```python
from build123d import *

# Parameters (mm, degrees)
SKETCH_1_W           = 100.9
SKETCH_1_H           = 40
SKETCH_1_R           = 1.5
EXTRUDE_1_DEPTH      = 6
SKETCH_6_W           = 100.9
SKETCH_6_H           = 10
EXTRUDE_2_DEPTH      = 6
SKETCH_2_W           = 60.5
SKETCH_2_H           = 15
CUT_EXTRUDE_1_DEPTH  = 10
SKETCH_3_R           = 1
CUT_EXTRUDE_2_DEPTH  = 10
SKETCH_4_R           = 1.5
CUT_EXTRUDE_3_DEPTH  = 10
SKETCH_5_R           = 1.5
CUT_EXTRUDE_4_DEPTH  = 10
SKETCH_7_W           = 4
SKETCH_7_H           = 15
CUT_EXTRUDE_5_DEPTH  = 6
CUT_EXTRUDE_6_DEPTH  = 6
FILLET_1_R           = 0.5
FILLET_2_R           = 1
SKETCH_9_W           = 100.9
SKETCH_9_H           = 15
EXTRUDE_3_DEPTH      = 6
SKETCH_10_W          = 16.5
SKETCH_10_H          = 15
CUT_EXTRUDE_7_DEPTH  = 6
SKETCH_11_W          = 6
SKETCH_11_H          = 15
EXTRUDE_4_DEPTH      = 20
SKETCH_12_R          = 2.5
CUT_EXTRUDE_8_DEPTH  = 6
SKETCH_13_R          = 1.5
CUT_EXTRUDE_9_DEPTH  = 6
SKETCH_14_R          = 1.5
CUT_EXTRUDE_10_DEPTH = 6
SKETCH_15_W          = 20
SKETCH_15_H          = 2
EXTRUDE_5_DEPTH      = 6
FILLET_4_R           = 2
FILLET_5_R           = 2
SKETCH_19_R          = 4.5
SKETCH_19_R_2        = 2.5
EXTRUDE_6_DEPTH      = 55.9


with BuildPart() as part:
    # 草图1 → 凸台-拉伸1 (new body)
    with BuildSketch(Plane.XY):
        with Locations((0, 10)):
            Rectangle(SKETCH_1_W, SKETCH_1_H)
        with Locations((42.3, 25)):
            Circle(SKETCH_1_R, mode=Mode.SUBTRACT)
        with Locations((42.3, 5)):
            Circle(SKETCH_1_R, mode=Mode.SUBTRACT)
        with Locations((35.3, 5)):
            Circle(SKETCH_1_R, mode=Mode.SUBTRACT)
        with Locations((35.3, -5)):
            Circle(SKETCH_1_R, mode=Mode.SUBTRACT)
        with Locations(Location((-35.3, -5, 0), (0, 0, 180))):
            Circle(SKETCH_1_R, mode=Mode.SUBTRACT)
        with Locations(Location((-35.3, 5, 0), (0, 0, 180))):
            Circle(SKETCH_1_R, mode=Mode.SUBTRACT)
        with Locations(Location((-42.3, 5, 0), (0, 0, 180))):
            Circle(SKETCH_1_R, mode=Mode.SUBTRACT)
        with Locations(Location((-42.3, 25, 0), (0, 0, 180))):
            Circle(SKETCH_1_R, mode=Mode.SUBTRACT)
    extrude(amount=EXTRUDE_1_DEPTH)

    # 草图6 → 凸台-拉伸2 (add)
    with BuildSketch(Plane.XY.offset(6)):
        with Locations((0, 35)):
            Rectangle(SKETCH_6_W, SKETCH_6_H)
    extrude(amount=-EXTRUDE_2_DEPTH)

    # 草图2 → 切除-拉伸1 (cut)
    with BuildSketch(Plane.XY.offset(6)):
        with Locations((0, -2.5)):
            Rectangle(SKETCH_2_W, SKETCH_2_H)
    extrude(amount=-CUT_EXTRUDE_1_DEPTH, mode=Mode.SUBTRACT)

    # 草图3 → 切除-拉伸2 (cut)
    with BuildSketch(Plane.XY.offset(6)):
        with Locations((-30.25, 5)):
            Circle(SKETCH_3_R)
        with Locations((30.25, 5)):
            Circle(SKETCH_3_R)
    extrude(amount=-CUT_EXTRUDE_2_DEPTH, mode=Mode.SUBTRACT)

    # 草图4 → 切除-拉伸3 (cut)
    with BuildSketch(Plane.XY.offset(6)):
        with Locations((31, 34.5)):
            Circle(SKETCH_4_R)
        with Locations((31, 24.5)):
            Circle(SKETCH_4_R)
        with Locations((-31, 24.5)):
            Circle(SKETCH_4_R)
        with Locations((-31, 34.5)):
            Circle(SKETCH_4_R)
    extrude(amount=-CUT_EXTRUDE_3_DEPTH, mode=Mode.SUBTRACT)

    # 草图5 → 切除-拉伸4 (cut)
    with BuildSketch(Plane.XY.offset(6)):
        with Locations((-15, 12.5)):
            Circle(SKETCH_5_R)
        with Locations((5, 12.5)):
            Circle(SKETCH_5_R)
    extrude(amount=-CUT_EXTRUDE_4_DEPTH, mode=Mode.SUBTRACT)

    # 草图7 → 切除-拉伸5 (cut)
    with BuildSketch(Plane.XY.offset(6)):
        with Locations((36, 27)):
            Rectangle(SKETCH_7_W, SKETCH_7_H)
        with Locations((-36, 27)):
            Rectangle(SKETCH_7_W, SKETCH_7_H)
    extrude(amount=-CUT_EXTRUDE_5_DEPTH, mode=Mode.SUBTRACT)

    # 草图8 → 切除-拉伸6 (cut)
    with BuildSketch(Plane.XY.offset(6)):
        with BuildLine():
            Line((-38, 33.5), (-38, 34.5))
            ThreePointArc((-38, 34.5), (-38.5, 34), (-38, 33.5))
        make_face()
        with BuildLine():
            Line((-34, 34.5), (-34, 33.5))
            ThreePointArc((-34, 33.5), (-33.5, 34), (-34, 34.5))
        make_face()
        with BuildLine():
            Line((-38, 19.5), (-38, 20.5))
            ThreePointArc((-38, 20.5), (-38.5, 20), (-38, 19.5))
        make_face()
        with BuildLine():
            Line((-34, 20.5), (-34, 19.5))
            ThreePointArc((-34, 19.5), (-33.5, 20), (-34, 20.5))
        make_face()
        with BuildLine():
            ThreePointArc((38, 33.5), (38.5, 34), (38, 34.5))
            Line((38, 34.5), (38, 33.5))
        make_face()
        with BuildLine():
            ThreePointArc((34, 34.5), (33.5, 34), (34, 33.5))
            Line((34, 33.5), (34, 34.5))
        make_face()
        with BuildLine():
            ThreePointArc((34, 20.5), (33.5, 20), (34, 19.5))
            Line((34, 19.5), (34, 20.5))
        make_face()
        with BuildLine():
            ThreePointArc((38, 19.5), (38.5, 20), (38, 20.5))
            Line((38, 20.5), (38, 19.5))
        make_face()
    extrude(amount=-CUT_EXTRUDE_6_DEPTH, mode=Mode.SUBTRACT)

    # 圆角1
    fillet_1_edges = [part.edges().sort_by_distance(p)[0] for p in [
        (38, 33.5, 3),
        (-34, 20.5, 3),
        (-38, 20.5, 3),
        (-34, 33.5, 3),
        (34, 33.5, 3),
        (34, 20.5, 3),
        (38, 20.5, 3),
        (-38, 33.5, 3),
    ]]
    fillet(fillet_1_edges, radius=FILLET_1_R)

    # 圆角2
    fillet_2_edges = [part.edges().sort_by_distance(p)[0] for p in [
        (-30.25, 4, 3),
        (30.25, 4, 3),
        (-29.25, 5, 3),
        (29.25, 5, 3),
    ]]
    fillet(fillet_2_edges, radius=FILLET_2_R)

    # 草图9 → 凸台-拉伸3 (add)
    with BuildSketch(Plane.XY.offset(6)):
        with Locations((0, 47.5)):
            Rectangle(SKETCH_9_W, SKETCH_9_H)
    extrude(amount=-EXTRUDE_3_DEPTH)

    # 草图10 → 切除-拉伸7 (cut)
    with BuildSketch(Plane.XY.offset(6)):
        with Locations((-42.2, 47.5)):
            Rectangle(SKETCH_10_W, SKETCH_10_H)
        with Locations((42.2, 47.5)):
            Rectangle(SKETCH_10_W, SKETCH_10_H)
    extrude(amount=-CUT_EXTRUDE_7_DEPTH, mode=Mode.SUBTRACT)

    # 草图13 → 切除-拉伸9 (cut)
    with BuildSketch(Plane.XY.offset(6)):
        with Locations((-25, 47)):
            Circle(SKETCH_13_R)
        with Locations((-25, 37)):
            Circle(SKETCH_13_R)
        with Locations((25, 37)):
            Circle(SKETCH_13_R)
        with Locations((25, 47)):
            Circle(SKETCH_13_R)
    extrude(amount=-CUT_EXTRUDE_9_DEPTH, mode=Mode.SUBTRACT)

    # 圆角5
    fillet_5_edges = [part.edges().sort_by_distance(p)[0] for p in [
        (50.45, 40, 3),
        (33.95, 40, 3),
        (33.95, 55, 3),
        (-33.95, 55, 3),
        (-33.95, 40, 3),
        (-50.45, 40, 3),
        (-30.25, -10, 3),
        (30.25, -10, 3),
        (50.45, -10, 3),
        (-50.45, -10, 3),
    ]]
    fillet(fillet_5_edges, radius=FILLET_5_R)


with BuildPart() as body_2:
    # 草图11 → 凸台-拉伸4 (new body)
    with BuildSketch(Plane.XY.offset(6)):
        with Locations((30.95, 47.5)):
            Rectangle(SKETCH_11_W, SKETCH_11_H)
    extrude(amount=EXTRUDE_4_DEPTH)

    # 草图12 → 切除-拉伸8 (cut)
    with BuildSketch(Plane(origin=(33.95, 0, 0), x_dir=(0, 0, -1), z_dir=(1, 0, 0))):
        with Locations((-21, 46.5)):
            Circle(SKETCH_12_R)
    extrude(amount=-CUT_EXTRUDE_8_DEPTH, mode=Mode.SUBTRACT)

    # 草图14 → 切除-拉伸10 (cut)
    with BuildSketch(Plane(origin=(33.95, 0, 0), x_dir=(0, 0, -1), z_dir=(1, 0, 0))):
        with Locations((-9, 42)):
            Circle(SKETCH_14_R)
        with Locations((-9, 52)):
            Circle(SKETCH_14_R)
    extrude(amount=-CUT_EXTRUDE_10_DEPTH, mode=Mode.SUBTRACT)

    # 草图15 → 凸台-拉伸5 (add)
    with BuildSketch(Plane(origin=(33.95, 0, 0), x_dir=(0, 0, -1), z_dir=(1, 0, 0))):
        with Locations((-16, 39)):
            Rectangle(SKETCH_15_W, SKETCH_15_H)
    extrude(amount=-EXTRUDE_5_DEPTH)

    # 圆角4
    fillet_4_edges = [body_2.edges().sort_by_distance(p)[0] for p in [
        (30.95, 55, 26),
        (30.95, 38, 26),
    ]]
    fillet(fillet_4_edges, radius=FILLET_4_R)


with BuildPart() as body_3:
    # 镜向1: mirrored copy
    add(body_2.part.mirror(Plane(origin=(0, 0, 0), x_dir=(0, 0, 1), z_dir=(1, 0, 0))))


with BuildPart() as body_4:
    # 草图19 → 凸台-拉伸6 (new body)
    with BuildSketch(Plane(origin=(-27.95, 0, 0), x_dir=(0, 0, -1), z_dir=(1, 0, 0))):
        with Locations(Location((-21, 46.5, 0), (0, 0, 180))):
            Circle(SKETCH_19_R)
        with Locations((-21, 46.5)):
            Circle(SKETCH_19_R_2, mode=Mode.SUBTRACT)
    extrude(amount=EXTRUDE_6_DEPTH)


solid = part.part
```
CAD build for the part. Positions are in the model's coordinates, mm. A direction names the side the tool comes from. Coordinates: 2 decimals unless noted, no trailing zeros. Order: outer loops, then holes, each group sorted by start corner. A loop starts at its lowest first (then second) coordinate and runs counter-clockwise, first axis right, second up. Notation, with made-up numbers: M 29.5,-35.75 L 75.5,-35.75 A35 ccw 75.5,3.25 Z; hole C -12,-14 d8. An arc over 180 degrees is marked long. Answer as CSV lines item,"result".
1) Mould opens along X. For faces 1 (the flat face through (50.45, 15, 3)), 2 (the cylindrical face through (-36.73, -5.45, 2.96)), 3 (the flat face through (0, 55, 3)) say: released by +X, released by -X, zero draft, split by the parting line, or undercut.
Verdict:
face 1,"released by +X"
face 2,"undercut"
face 3,"zero draft"
2) Flat gauge pins, fed straight in: P1, Ø1.6, axis at x = 30.25, y = 5, coming from the +Z side; P2, Ø5, axis at x = 25, y = 37, coming from the +Z side; P3, Ø3, axis at y = 47, z = 3, coming from the +X side; P4, Ø3, axis at x = -36.5, z = 3.5, coming from the +Y side. Where does each tip first touch, or does it go through?
Verdict:
P1,"through"
P2,"z = 6"
P3,"x = 33.95"
P4,"y = 40.24"
3) Cut at A-A (y = -5). List the corners of the cut face in (x, z), then the cut area to 3 significant figures.
Verdict:
outline,"M -50.45,0 L -36.8,0 L -36.8,6 L -50.45,6 Z; M -33.8,0 L -30.25,0 L -30.25,6 L -33.8,6 Z; M 30.25,0 L 33.8,0 L 33.8,6 L 30.25,6 Z; M 36.8,0 L 50.45,0 L 50.45,6 L 36.8,6 Z"
area,"206 mm2"
4) 3-axis set-ups, long thin cutter, end or side, ignore diameter. For faces 4 (the flat face through (38, 27, 3)), 5 (the cylindrical face through (-33.38, 54.4, 2.96)), 6 (the flat face through (0, 5, 3)): which of +Z, -Z, +X, -X, +Y, -Y reach the whole face in a straight line?
Verdict:
face 4,"+Z, -Z"
face 5,"+Z, -Z, -X, +Y"
face 6,"+Z, -Z, -Y"
5) Drill centre lines: L1, parallel to X at y = 29, z = 5.35; L2, parallel to Y at x = -25, z = 4.7; L3, parallel to Y at x = -36, z = 4.9. Where is each one in solid material? Low to high. Write a range as from..to.
Verdict:
L1,"-50.45..-38, -34..34, 38..50.45"
L2,"5..35.5, 38.5..45.5, 48.5..55"
L3,"-10..-6.33, -3.67..3.67, 6.33..19.5, 34.5..40"
6) Cut at B-B (x = -15). List the corners of the cut face in (y, z).
Verdict:
outline,"M 5,0 L 11,0 L 11,6 L 5,6 Z; M 14,0 L 55,0 L 55,6 L 14,6 Z"
7) Cut at C-C (x = 42.3). List the corners of the cut face in (y, z), then the cut area to 3 significant figures.
Verdict:
outline,"M -10,0 L 3.5,0 L 3.5,6 L -10,6 Z; M 6.5,0 L 23.5,0 L 23.5,6 L 6.5,6 Z; M 26.5,0 L 40,0 L 40,6 L 26.5,6 Z"
area,"264 mm2"
8) Cut at D-D (z = 1.4). Give the number of separate pieces and of enclosed holes in the cut face, then the cut area to 3 significant figures.
Verdict:
separate pieces,"1"
enclosed holes,"20"
area,"4,900 mm2"
